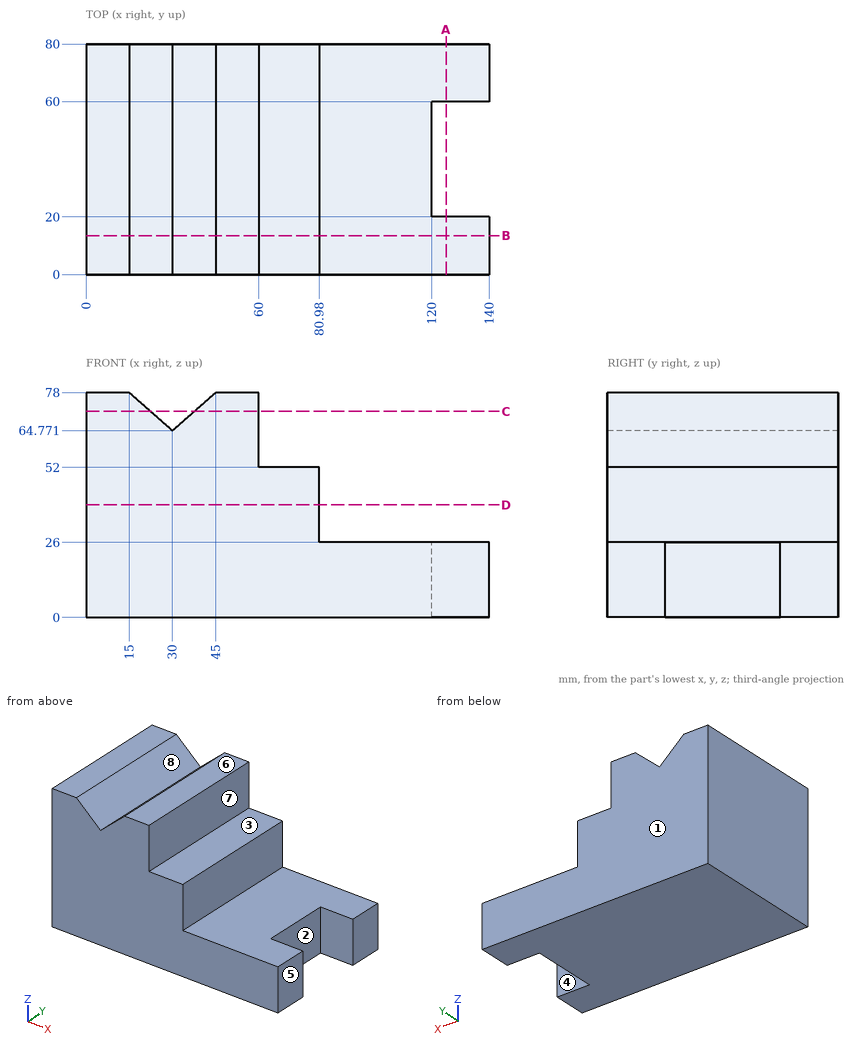
Part print with two shaded views. Sizes in mm from the minimum x, y, z corner. A direction names the side the tool comes from. Round coordinates to 2 decimals unless told otherwise and drop trailing zeros. Loops run counter-clockwise (first coordinate to the right, second up) from the corner with the lowest first, then second, coordinate; pieces in that order, holes last.
Item 1: Saw through at D-D (z = 39). List the corners of the cut face in (x, y), then the cut area to 3 significant figures.
Item 2: Two-plate mould, pull along Y, no slides. Class the marked faces 1, 2 and 3: released by +Y, released by -Y, zero draft, split by the parting line, or undercut.
Item 3: Saw through at C-C (z = 71.5). List the corners of the cut face in (x, y), then the cut area to 3 significant figures.
Item 4: Saw through at B-B (y = 13.5). List the corners of the cut face in (x, z).
Item 5: Drill centre lines: line 1 along Z through (x, y) = (66, 25.5); line 2 along Y through (x, z) = (128, 17.5); line 3 along X through (y, z) = (36.5, 58). Where is each one in solid material? Low to high.
Item 6: Which spindle directions (+Z, -Z, +X, -X, +Y, -Y) get a long thin tool onto all of the face, cutting with end or side? Do the marked faces 4, 5, 6, 7 and 8. Say none if no direction does.
Item 7: Pin check, flat tips, straight feed: P1, Ø8, axis at y = 30, z = 16, coming from the +X side; P2, Ø1.5, axis at x = 101, z = 10, coming from the -Y side; P3, Ø17.5, axis at x = 116.5, y = 41, coming from the +Z side; P4, Ø21, axis at y = 53, z = 44.5, coming from the +X side. Stop position of each tip, or through.
Item 8: Saw through at A-A (x = 125). List the corners of the cut face in (y, z).
Worked answers:
1. outline: (0, 0) - (80.98, 0) - (80.98, 80) - (0, 80) - close
1. area: 6,480 mm2
2. face 1: released by +Y
2. face 2: undercut
2. face 3: zero draft
3. outline: (0, 0) - (22.37, 0) - (22.37, 80) - (0, 80) - close; (37.63, 0) - (60, 0) - (60, 80) - (37.63, 80) - close
3. area: 3,580 mm2
4. outline: (0, 0) - (140, 0) - (140, 26) - (80.98, 26) - (80.98, 52) - (60, 52) - (60, 78) - (45, 78) - (30, 64.77) - (15, 78) - (0, 78) - close
5. line 1: z = 0 to 52
5. line 2: y = 0 to 20, 60 to 80
5. line 3: x = 0 to 60
6. face 4: +Z, -Z, +X
6. face 5: +Z, -Z, +X, +Y, -Y
6. face 6: +Z, +X, -X, +Y, -Y
6. face 7: +Z, +X, +Y, -Y
6. face 8: +Z, +Y, -Y
7. P1: stops at x = 120
7. P2: stops at y = 0
7. P3: stops at z = 26
7. P4: stops at x = 80.98
8. outline: (0, 0) - (20, 0) - (20, 26) - (0, 26) - close; (60, 0) - (80, 0) - (80, 26) - (60, 26) - close
